The listing builds one solid part. Answer for the finished solid, in the listing's coordinates (mm). A direction names the side the tool comes from. Give positions to 0.01 mm unless a question says otherwise; leave off trailing zeros. Loops run counter-clockwise (first coordinate to the right, second up) from the corner with the lowest first, then second, coordinate; pieces in that order, holes last. Notation, with made-up numbers: (15, -39) - (21, -39) arc R22 cw to (21, -11) - close; hole circle Ø9 at (-12, -22). An arc over 180 degrees is marked (long way). Write item = value, one per line. Start each with the question number.
1) The part is cut by section B-B on x = 6. Write down the section's boundary in (y, z), plus the area to 3 significant figures.
2) Which of the six approach directions +Z, -Z, +X, -X, +Y, -Y give full straight-line access (tool end or side, diameter ignored) to faces 1 (the cylindrical face through (43.133, 60.037, 0.986)), 2 (the flat face through (24, 101, 3))?
3) The part is cut by section A-A on y = 142. Write down the section's boundary in (x, z), plus the area to 3 significant figures.
4) The mould has two halves that part along Y. Classify faces 3 (the flat face through (24, 148, 1)), 4 (the cylindrical face through (24.296, 145.074, 0.986)), 5 (the flat face through (0, 99, 1)), 6 (the flat face through (24, 52, 1)): +Y half, -Y half, draft (parallel to the pull), parting line (faces both ways), or undercut.
5) The part is cut by section C-C on y = 58. Write down the section's boundary in (x, z), plus the area to 3 significant figures.
6) Consider probe 1 along Y at (x, z) = (25, 1.95); probe 2 along X at (y, z) = (142, 0.75); probe 3 along Y at (x, z) = (6, 1.3). Determine where each line is inside the solid, lowest interval first.
7) A flat-ended cylindrical pin translates along its axis: P1, Ø2, axis at x = 43.5, y = 58, coming from the -Z side. Find the tip coordinate at first contact, or state that the pin passes through.
from build123d import *

# Parameters (mm, degrees)
SKETCH_W      = 49.4
SKETCH_H      = 96
PAD_DEPTH     = 3
SKETCH001_R   = 3.1
SKETCH001_R_2 = 2.674465
SKETCH001_R_3 = 2.054582
POCKET_DEPTH  = 2


with BuildPart() as part:
    # Sketch → Pad (new body)
    with BuildSketch(Plane.XY):
        with Locations((24.7, 100)):
            Rectangle(SKETCH_W, SKETCH_H)
    extrude(amount=PAD_DEPTH)

    # Sketch001 → Pocket (cut)
    with BuildSketch(Plane.XY):
        with Locations((24.7, 142)):
            Circle(SKETCH001_R)
        with Locations((6, 58)):
            Circle(SKETCH001_R_2)
        with Locations((43.4, 58)):
            Circle(SKETCH001_R_3)
    extrude(amount=POCKET_DEPTH, mode=Mode.SUBTRACT)


solid = part.part
Answer below:
q1.outline = (52, 0) - (55.33, 0) - (55.33, 2) - (60.67, 2) - (60.67, 0) - (148, 0) - (148, 3) - (52, 3) - close
q1.area = 277 mm2
q2.face_1 = -Z
q2.face_2 = +Z, +X, -X, +Y, -Y
q3.outline = (0, 0) - (21.6, 0) - (21.6, 2) - (27.8, 2) - (27.8, 0) - (49.4, 0) - (49.4, 3) - (0, 3) - close
q3.area = 136 mm2
q4.face_3 = +Y half
q4.face_4 = undercut
q4.face_5 = draft
q4.face_6 = -Y half
q5.outline = (0, 0) - (3.33, 0) - (3.33, 2) - (8.67, 2) - (8.67, 0) - (41.35, 0) - (41.35, 2) - (45.45, 2) - (45.45, 0) - (49.4, 0) - (49.4, 3) - (0, 3) - close
q5.area = 129 mm2
q6.probe_1 = 52 to 138.91, 145.09 to 148
q6.probe_2 = 0 to 21.6, 27.8 to 49.4
q6.probe_3 = 52 to 55.33, 60.67 to 148
q7.P1 = 2
